Input: part model. Units: mm. Frame: model coordinates. Give positions to 0.01 mm unless a question says otherwise; leave off trailing zeros. Order: outer loops, then holes, each group sorted by start corner. A loop starts at its lowest first (then second) coordinate and runs counter-clockwise, first axis right, second up. Notation, with made-up numbers: (-29.5, 23.25) - (-8.5, 23.25) arc R32 ccw to (-8.5, 58.25) - close; hole circle Ø6 at (10.5, 36.5). An arc over 180 degrees is marked (long way). Answer in a Markdown table with one row per item. Add a question column.
1. Section query A-A on x = 0. Return loops of the section in (y, z) (3 decimals), and give its area (3 significant figures).
2. Section query B-B on z = 0. Return loops of the section in (x, y) (3 decimals), and give its area (3 significant figures).
3. Ray query, line 1 (X direction, y = 2.5, z = 0); line 2 (X direction, y = 3.5, z = -56.5); line 3 (X direction, y = 2.5, z = 15). Return the intervals inside material, ascending. Write a range as [from, to].
4. Mould query, pull axis Z, two halves, no side actions, for faces 1 (the face through (-41.09, 4.83, 43.26)), 2 (the face through (50, 0, -16)), 3 (the face through (46.367, 4.696, 60.47)). Classes: released by +Z, released by -Z, zero draft, split by the parting line, or undercut.
5. Section query C-C on x = -21. Return loops of the section in (y, z) (3 decimals), and give its area (3 significant figures).
6. Section query D-D on z = 65. Return loops of the section in (x, y) (3 decimals), and give its area (3 significant figures).
7. Contact query for flat-ended pins moving along their axis: pin 1 (4.5 mm diameter, centred on x = 56.84, z = 15.23, fed in from -Y); pin 2 (3 mm diameter, centred on x = -15.23, z = 56.84, fed in from +Y); pin 3 (1 mm diameter, centred on y = 7.5, z = 16, fed in from -X); pin 4 (2 mm diameter, centred on x = -21.5, y = 7, fed in from -Z). Output: stop coordinate, or through.
```python
from build123d import *

# Parameters (mm, degrees)
SKETCH1_R           = 76.2
SKETCH1_R_2         = 51.1048
BOSS_EXTRUDE1_DEPTH = 9.525
SKETCH2_R           = 1.7272
CUT_EXTRUDE1_DEPTH  = 109.183203987
SKETCH3_R           = 6.249999946
CUT_EXTRUDE2_DEPTH  = 109.183203987


with BuildPart() as part:
    # Sketch1 → Boss-Extrude1 (new body)
    with BuildSketch(Plane(origin=(0, 0, 0), x_dir=(1, 0, 0), z_dir=(0, 1, 0))):
        with Locations(Location((0, 0, 0), (0, 0, 90))):
            Circle(SKETCH1_R)
        with Locations(Location((0, 0, 0), (0, 0, 90))):
            Circle(SKETCH1_R_2, mode=Mode.SUBTRACT)
    extrude(amount=BOSS_EXTRUDE1_DEPTH)

    # Sketch2 → Cut-Extrude1 (cut, through all)
    with BuildSketch(Plane(origin=(0, 9.525, 0), x_dir=(1, 0, 0), z_dir=(0, 1, 0))):
        with Locations(Location((-15.231500779, 56.844734782, 0), (0, 0, 270))):
            Circle(SKETCH2_R)
        with Locations(Location((15.231500779, 56.844734782, 0), (0, 0, 270))):
            Circle(SKETCH2_R)
        with Locations(Location((41.613234004, 41.613234004, 0), (0, 0, 270))):
            Circle(SKETCH2_R)
        with Locations(Location((56.844734782, 15.231500779, 0), (0, 0, 270))):
            Circle(SKETCH2_R)
        with Locations(Location((56.844734782, -15.231500779, 0), (0, 0, 270))):
            Circle(SKETCH2_R)
        with Locations(Location((41.613234004, -41.613234004, 0), (0, 0, 270))):
            Circle(SKETCH2_R)
        with Locations(Location((15.231500779, -56.844734782, 0), (0, 0, 270))):
            Circle(SKETCH2_R)
        with Locations(Location((-15.231500779, -56.844734782, 0), (0, 0, 270))):
            Circle(SKETCH2_R)
        with Locations(Location((-41.613234004, -41.613234004, 0), (0, 0, 270))):
            Circle(SKETCH2_R)
        with Locations(Location((-56.844734782, -15.231500779, 0), (0, 0, 270))):
            Circle(SKETCH2_R)
        with Locations(Location((-56.844734782, 15.231500779, 0), (0, 0, 270))):
            Circle(SKETCH2_R)
        with Locations(Location((-41.613234004, 41.613234004, 0), (0, 0, 270))):
            Circle(SKETCH2_R)
    extrude(amount=-CUT_EXTRUDE1_DEPTH, mode=Mode.SUBTRACT)

    # Sketch3 → Cut-Extrude2 (cut, through all)
    with BuildSketch(Plane(origin=(0, 9.525, 0), x_dir=(1, 0, 0), z_dir=(0, 1, 0))):
        with Locations(Location((-62.85000003, 0, 0), (0, 0, 270))):
            Circle(SKETCH3_R)
        with Locations(Location((0, 62.85000003, 0), (0, 0, 270))):
            Circle(SKETCH3_R)
        with Locations(Location((62.85000003, 0, 0), (0, 0, 270))):
            Circle(SKETCH3_R)
        with Locations(Location((0, -62.85000003, 0), (0, 0, 270))):
            Circle(SKETCH3_R)
    extrude(amount=-CUT_EXTRUDE2_DEPTH, mode=Mode.SUBTRACT)


solid = part.part
```
Answer:
| question | item | result |
|---|---|---|
| 1 | outline | (0, -76.2) - (9.525, -76.2) - (9.525, -69.1) - (0, -69.1) - close; (0, -56.6) - (9.525, -56.6) - (9.525, -51.105) - (0, -51.105) - close; (0, 51.105) - (9.525, 51.105) - (9.525, 56.6) - (0, 56.6) - close; (0, 69.1) - (9.525, 69.1) - (9.525, 76.2) - (0, 76.2) - close |
| 1 | area | 240 mm² |
| 2 | outline | (-76.2, 0) - (-69.1, 0) - (-69.1, 9.525) - (-76.2, 9.525) - close; (-56.6, 0) - (-51.105, 0) - (-51.105, 9.525) - (-56.6, 9.525) - close; (51.105, 0) - (56.6, 0) - (56.6, 9.525) - (51.105, 9.525) - close; (69.1, 0) - (76.2, 0) - (76.2, 9.525) - (69.1, 9.525) - close |
| 2 | area | 240 mm² |
| 3 | line 1 | x = [-76.2, -69.1], [-56.6, -51.1], [51.1, 56.6], [69.1, 76.2] |
| 3 | line 2 | x = [-51.13, -16.92], [-13.54, 13.54], [16.92, 51.13] |
| 3 | line 3 | x = [-74.71, -58.56], [-55.13, -48.85], [48.85, 55.13], [58.56, 74.71] |
| 4 | face 1 | undercut |
| 4 | face 2 | zero draft |
| 4 | face 3 | split by the parting line |
| 5 | outline | (0, -73.249) - (9.525, -73.249) - (9.525, -46.591) - (0, -46.591) - close; (0, 46.591) - (9.525, 46.591) - (9.525, 73.249) - (0, 73.249) - close |
| 5 | area | 508 mm² |
| 6 | outline | (-39.767, 0) - (-5.869, 0) - (-5.869, 9.525) - (-39.767, 9.525) - close; (5.869, 0) - (39.767, 0) - (39.767, 9.525) - (5.869, 9.525) - close |
| 6 | area | 646 mm² |
| 7 | pin 1 | stops at y = 0 |
| 7 | pin 2 | passes through |
| 7 | pin 3 | stops at x = -74.61 |
| 7 | pin 4 | stops at z = -73.39 |
